Can you work these out from the model? Positions are in its coordinate system, mm. Face numbers are marked on the shaded views. A direction names the side the tool comes from. Give positions to 0.01 mm unless a question says otherwise; leave off trailing zeros. Order: outer loops, then holes, each group sorted by start corner. A loop starts at its lowest first (then second) coordinate and runs counter-clockwise, first axis right, second up.
Item 1: I want a section at A-A, the plane z = 0. Count the separate pieces of the cut face and the enclosed holes in it, then the cut area to 3 significant figures.
Item 2: I'm going to push flat-ended pins straight in: pin 1 Ø4 at (y, z) = (32.5, 1.5) entering from +X; pin 2 Ø10 at (x, y) = (-2, 48) entering from -Z; pin 3 Ø6 at (y, z) = (46.5, -2.5) entering from -X; pin 4 Ø1.9 at (x, z) = (-12.7, 0) entering from -Y. Where does each tip first touch, or does it pass through?
Item 3: If I drill on line 1 along X through (y, z) = (99.3, 0); line 2 along Y through (x, z) = (15, 2.5); line 3 along Z through (x, y) = (12.7, 100.1), over which ranges is the centre line in solid material (lowest first)?
Item 4: Which directions (+Z, -Z, +X, -X, +Y, -Y) give clear straight access to the entire face, cutting with the end or side of a thin tool? Please do the marked faces 1, 2, 3, 4 and 5.
Item 5: If we mould it in two halves opening along Y, with no side actions, what happens to the marked faces 6, 7 and 8? For each: +Y half, -Y half, draft (parallel to the pull), parting line (faces both ways), or undercut.
Item 6: I want a section at B-B, the plane x = -12.7. Write out the boundary of the cut face in (y, z), then the cut area to 3 significant figures.
Item 7: I want a section at D-D, the plane y = 54.5. Write out the boundary of the cut face in (x, z), then the cut area to 3 significant figures.
Item 8: I want a section at C-C, the plane z = -5. Write out the boundary of the cut face in (x, y), then the cut area to 3 significant figures.
```python
from build123d import *

# Parameters (mm, degrees)
BOSS_EXTRUDE1_DEPTH = 6.35
SKETCH2_R           = 1.5875
MOUNT_HOLES_DEPTH   = 12.7
FILLET1_R           = 2.54
CUT_EXTRUDE1_DEPTH  = 105.599497571
FILLET2_R           = 2.54


with BuildPart() as part:
    # Sketch1 → Boss-Extrude1 (new, symmetric)
    with BuildSketch(Plane.XY):
        Polygon((19.05, 0), (-19.05, 0), (-19.05, 3.81), (-6.35, 3.81), (-6.35, 97.4598), (-19.05, 97.4598), (-19.05, 101.2698), (19.05, 101.2698), (19.05, 97.4598), (6.35, 97.4598), (6.35, 3.81), (19.05, 3.81), align=None)
    extrude(amount=BOSS_EXTRUDE1_DEPTH, both=True)

    # Sketch2 → Mount_Holes (cut)
    with BuildSketch(Plane(origin=(0, 3.81, 0), x_dir=(1, 0, 0), z_dir=(0, 1, 0))):
        with Locations(Location((12.7, 0, 0), (0, 0, 180))):
            Circle(SKETCH2_R)
        with Locations(Location((-12.7, 0, 0), (0, 0, 180))):
            Circle(SKETCH2_R)
    mount_holes = extrude(amount=-MOUNT_HOLES_DEPTH, mode=Mode.SUBTRACT)

    # Mirror1: Mount_Holes across plane
    add(mount_holes.mirror(Plane.ZX.offset(50.6349)), mode=Mode.SUBTRACT)

    # Fillet1
    fillet1_edges = [part.edges().sort_by_distance(p)[0] for p in [
        (-6.35, 3.81, 0),
        (-6.35, 97.4598, 0),
        (6.35, 97.4598, 0),
        (6.35, 3.81, 0),
    ]]
    fillet(fillet1_edges, radius=FILLET1_R)

    # Sketch3 → Cut-Extrude1 (cut, through all)
    with BuildSketch(Plane.ZY.offset(6.35)):
        Polygon((-6.35, 25.2349), (-6.35, 76.0349), (-1.27, 63.3349), (-1.27, 37.9349), align=None)
    extrude(amount=-CUT_EXTRUDE1_DEPTH, mode=Mode.SUBTRACT)

    # Fillet2
    fillet2_edges = [part.edges().sort_by_distance(p)[0] for p in [
        (0, 25.2349, -6.35),
        (0, 76.0349, -6.35),
        (0, 63.3349, -1.27),
        (0, 37.9349, -1.27),
    ]]
    fillet(fillet2_edges, radius=FILLET2_R)


solid = part.part
```
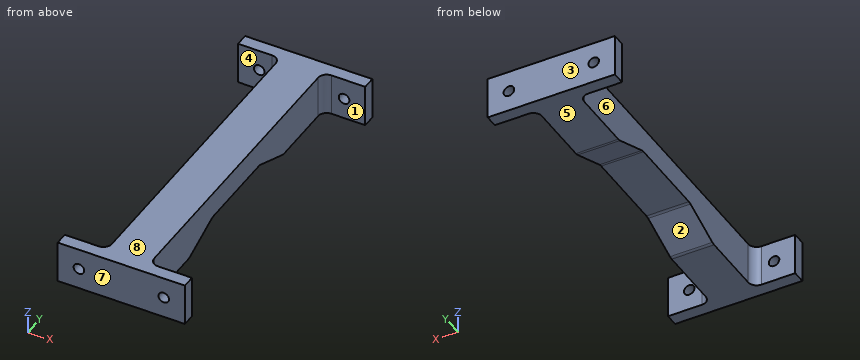
Results list:
1. separate pieces: 5
1. enclosed holes: 0
1. area: 1,440 mm2
2. pin 1: stops at x = 6.35
2. pin 2: stops at z = -1.27
2. pin 3: stops at x = -6.35
2. pin 4: passes through
3. line 1: x = -19.05 to -14.29, -11.11 to 11.11, 14.29 to 19.05
3. line 2: y = 0 to 3.81, 97.46 to 101.27
3. line 3: z = -6.35 to -1.59, 1.59 to 6.35
4. face 1: +Z, -Z, +X
4. face 2: -Z, +X, -X
4. face 3: +Z, -Z, +X, -X, +Y
4. face 4: +Z, -Z, -X
4. face 5: -Z, +X, -X, +Y, -Y
5. face 6: undercut
5. face 7: -Y half
5. face 8: draft
6. outline: (0, -6.35) - (3.81, -6.35) - (3.81, -1.59) - (0, -1.59) - close; (0, 1.59) - (3.81, 1.59) - (3.81, 6.35) - (0, 6.35) - close; (97.46, -6.35) - (101.27, -6.35) - (101.27, -1.59) - (97.46, -1.59) - close; (97.46, 1.59) - (101.27, 1.59) - (101.27, 6.35) - (97.46, 6.35) - close
6. area: 72.6 mm2
7. outline: (-6.35, -1.27) - (6.35, -1.27) - (6.35, 6.35) - (-6.35, 6.35) - close
7. area: 96.8 mm2
8. outline: (-19.05, 0) - (19.05, 0) - (19.05, 3.81) - (8.89, 3.81) arc R2.54 cw to (6.35, 6.35) - (6.35, 28.61) - (-6.35, 28.61) - (-6.35, 6.35) arc R2.54 cw to (-8.89, 3.81) - (-19.05, 3.81) - close; (-19.05, 97.46) - (-8.89, 97.46) arc R2.54 cw to (-6.35, 94.92) - (-6.35, 72.66) - (6.35, 72.66) - (6.35, 94.92) arc R2.54 cw to (8.89, 97.46) - (19.05, 97.46) - (19.05, 101.27) - (-19.05, 101.27) - close
8. area: 926 mm2
